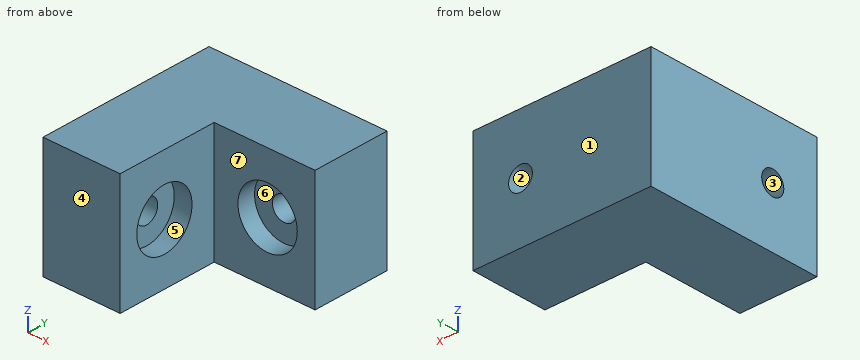
from build123d import *

# Parameters (mm, degrees)
F1_DEPTH = 20
F2_R     = 5
F3_DEPTH = 3
F4_R     = 2
F5_DEPTH = 10


# Not quite as in the source:
# - a pattern or mirror of a feature is missing from the dataset's text; its kind, count and spacing are read off the source's solid


with BuildPart() as f1:
    # F0 (on Top) → F1 (new body)
    with BuildSketch(Plane.XY):
        Polygon((30, 0), (0, 0), (0, -30), (13, -30), (13, -13), (30, -13), align=None)
    extrude(amount=F1_DEPTH)

    # F2 (on face) → F3 (cut)
    with BuildSketch(Plane.XZ.offset(13)):
        with Locations((22, 10)):
            Circle(F2_R)
    f3 = extrude(amount=-F3_DEPTH, mode=Mode.SUBTRACT)

    # F3_copies: F3 across plane
    add(f3.mirror(Plane(origin=(0, 0, 0), x_dir=(0.7071067812, -0.7071067812, 0), z_dir=(-0.7071067812, -0.7071067812, 0))), mode=Mode.SUBTRACT)

    # F4 (on face) → F5 (cut, through all)
    with BuildSketch(Plane.XZ.offset(10)):
        with Locations((22, 10)):
            Circle(F4_R)
    f5 = extrude(amount=-F5_DEPTH, mode=Mode.SUBTRACT)

    # F5_copies: F5 across plane
    add(f5.mirror(Plane(origin=(0, 0, 0), x_dir=(-0.7071067812, 0.7071067812, 0), z_dir=(-0.7071067812, -0.7071067812, 0))), mode=Mode.SUBTRACT)


solid = f1.part
Could you check a few things on this model? Use its own coordinates, in mm. Face numbers are marked on the shaded views. A direction names the side the tool comes from. Round coordinates to 2 decimals unless told otherwise and drop trailing zeros. Order: outer loops, then holes, each group sorted by start corner. A loop starts at its lowest first (then second) coordinate and runs counter-clockwise, first axis right, second up.
Q1. Imagine slicing it at B-B, the plane z = 10. List the corners of the cut face in (x, y) for me.
Geometry says:
outline: (0, -30) - (13, -30) - (13, -27) - (10, -27) - (10, -24) - (0, -24) - close; (0, -20) - (10, -20) - (10, -17) - (13, -17) - (13, -13) - (17, -13) - (17, -10) - (20, -10) - (20, 0) - (0, 0) - close; (24, -10) - (27, -10) - (27, -13) - (30, -13) - (30, 0) - (24, 0) - close
Q2. Imagine slicing it at C-C, the plane y = -22. List the corners of the cut face in (x, z) for me.
Geometry says:
outline: (0, 0) - (13, 0) - (13, 5) - (10, 5) - (10, 8) - (0, 8) - close; (0, 12) - (10, 12) - (10, 15) - (13, 15) - (13, 20) - (0, 20) - close
Q3. Please list where these lines run through material, in increasing order: probe 1 along Z at (x, y) = (7.75, -22); probe 2 along Z at (x, y) = (11.6, -22); probe 3 along Y at (x, z) = (18.5, 8).
Geometry says:
probe 1: z = 0 to 8, 12 to 20
probe 2: z = 0 to 5, 15 to 20
probe 3: y = -10 to 0
Q4. Thinking about a two-plate mould opening in Y: for the marked faces 1, 2 and 3, which applies, released by +Y, released by -Y, zero draft, split by the parting line, or undercut?
Geometry says:
face 1: released by +Y
face 2: zero draft
face 3: undercut
Q5. I'm going to push flat-ended pins straight in: P1, Ø12, axis at x = 6, y = -6, coming from the -Z side; P2, Ø9, axis at x = 22, z = 10, coming from the -Y side; P3, Ø5, axis at x = 20, z = 14.5, coming from the -Y side; P4, Ø8, axis at y = -22.5, z = 12, coming from the +X side. Where does each tip first touch, or does it pass through?
Geometry says:
P1: stops at z = 0
P2: stops at y = -10
P3: stops at y = -13
P4: stops at x = 13
Q6. Imagine slicing it at D-D, the plane x = 8. List the corners of the cut face in (y, z) for me.
Geometry says:
outline: (-30, 0) - (0, 0) - (0, 20) - (-30, 20) - close; hole circle Ø4 at (-22, 10)
Q7. Imagine slicing it at A-A, the plane x = 22. List the corners of the cut face in (y, z) for me.
Geometry says:
outline: (-13, 0) - (0, 0) - (0, 8) - (-10, 8) - (-10, 5) - (-13, 5) - close; (-13, 15) - (-10, 15) - (-10, 12) - (0, 12) - (0, 20) - (-13, 20) - close
Q8. Which directions (+Z, -Z, +X, -X, +Y, -Y) give clear straight access to the entire face, cutting with the end or side of a thin tool? Please do the marked faces 4, 5, 6 and 7.
Geometry says:
face 4: +Z, -Z, +X, -X, -Y
face 5: +X
face 6: -Y
face 7: +Z, -Z, +X, -Y
